Here's how the part is built. I have some questions about the finished solid (model axes, mm). A direction names the side the tool comes from. Coordinates: 2 decimals unless noted, no trailing zeros. Write each loop counter-clockwise with the first axis right and the second up, starting at its lowest first coordinate (ties: lowest second). Pieces come first, ordered by that corner, then holes. Notation, with made-up numbers: (49, 51) -> (56, 51) arc R34 ccw to (56, 89) -> close; hole circle Ø9 at (74, -4.75). An arc over 180 degrees is marked (long way). Put each result on its own line as item: value. Start each with the question number.
Item 1: For pin 1 (1 mm diameter, centred on x = 38.5, z = 2.5, fed in from +Y); pin 2 (4 mm diameter, centred on x = -65.78, y = 65.78, fed in from +Z); pin 3 (2.5 mm diameter, centred on x = -65.78, y = -65.78, fed in from -Z); pin 4 (1.5 mm diameter, centred on y = -14, z = 3.5, fed in from +X), each with a flat end and sliding along its axis, tell me the tip position at first contact or that it passes through.
Item 2: If we mould it in two halves opening along Y, with no side actions, what happens to faces 5 (the face through (-25, 0, 2)), 6 (the face through (51.35, 58.42, 2.46)), 7 (the face through (76.44, -76.34, 2.46))? For each: released by +Y, released by -Y, zero draft, split by the parting line, or undercut.
Item 3: I want a section at A-A, the plane x = 4. List the corners of the cut face in (y, z) for me.
Item 4: I want a section at C-C, the plane z = 0.95. State how many separate pieces and enclosed holes the cut face has, then the cut area to 3 significant figures.
Item 5: On a 3-axis mill with a long thin cutter (end or side, diameter ignored), from which of +Z, -Z, +X, -X, +Y, -Y can I reach the whole of each face in a straight line? I mean faces 1 (the face through (-59.01, -51.94, 2.46)), 2 (the face through (59.01, 51.94, 2.46)), 3 (the face through (0, -37.5, 2)), 4 (the face through (0, 37.5, 2)). Say none if no direction works.
Item 6: I need wall thicknesses on line 1 (X direction, y = 22, z = 4.6); line 2 (X direction, y = -58.5, z = 1.8). Which ranges of each line are inside material? Lowest first, please. Write a range as [from, to].
from build123d import *

# Parameters (mm, degrees)
SKETCH1_R           = 1.5
SKETCH1_W           = 50
SKETCH1_H           = 50
BOSS_EXTRUDE1_DEPTH = 5


with BuildPart() as part:
    # Sketch1 → Boss-Extrude1 (new body)
    with BuildSketch(Plane.XY):
        Polygon((-79.926406871, -72.855339059), (-37.5, -30.428932188), (-37.5, 30.428932188), (-79.926406871, 72.855339059), (-72.855339059, 79.926406871), (-30.428932188, 37.5), (30.428932188, 37.5), (72.855339059, 79.926406871), (79.926406871, 72.855339059), (37.5, 30.428932188), (37.5, -30.428932188), (79.926406871, -72.855339059), (72.855339059, -79.926406871), (30.428932188, -37.5), (-30.428932188, -37.5), (-72.855339059, -79.926406871), align=None)
        with Locations((72.855339059, 72.855339059)):
            Circle(SKETCH1_R, mode=Mode.SUBTRACT)
        with Locations((65.784271247, 65.784271247)):
            Circle(SKETCH1_R, mode=Mode.SUBTRACT)
        with Locations(Location((-65.784271247, 65.784271247, 0), (0, 0, 180))):
            Circle(SKETCH1_R, mode=Mode.SUBTRACT)
        with Locations(Location((-72.855339059, 72.855339059, 0), (0, 0, 180))):
            Circle(SKETCH1_R, mode=Mode.SUBTRACT)
        with Locations(Location((72.855339059, -72.855339059, 0), (0, 0, 180))):
            Circle(SKETCH1_R, mode=Mode.SUBTRACT)
        with Locations(Location((65.784271247, -65.784271247, 0), (0, 0, 180))):
            Circle(SKETCH1_R, mode=Mode.SUBTRACT)
        with Locations((-72.855339059, -72.855339059)):
            Circle(SKETCH1_R, mode=Mode.SUBTRACT)
        with Locations((-65.784271247, -65.784271247)):
            Circle(SKETCH1_R, mode=Mode.SUBTRACT)
        Rectangle(SKETCH1_W, SKETCH1_H, mode=Mode.SUBTRACT)
    extrude(amount=BOSS_EXTRUDE1_DEPTH)


solid = part.part
Calculated:
1. pin 1: stops at y = 46.07
1. pin 2: stops at z = 5
1. pin 3: passes through
1. pin 4: stops at x = 37.5
2. face 5: undercut
2. face 6: released by +Y
2. face 7: released by -Y
3. outline: (-37.5, 0) -> (-25, 0) -> (-25, 5) -> (-37.5, 5) -> close; (25, 0) -> (37.5, 0) -> (37.5, 5) -> (25, 5) -> close
4. separate pieces: 1
4. enclosed holes: 9
4. area: 5,370 mm2
5. face 1: +Z, -Z, -X
5. face 2: +Z, -Z, +X
5. face 3: +Z, -Z, -Y
5. face 4: +Z, -Z, +Y
6. line 1: x = [-37.5, -25], [25, 37.5]
6. line 2: x = [-65.57, -51.43], [51.43, 65.57]
